Answer from the drawing. Dimensions are ordinates in mm from the lowest x, y and z of the part. Give positions to 0.01 mm unless a question says otherwise; leave off trailing zeros. Loops run counter-clockwise (first coordinate to the right, second up) from the corner with the lowest first, then second, coordinate; pieces in that order, holes last. Notation, with made-up numbers: (8.5, 10.25) -> (29.5, 10.25) arc R24 cw to (29.5, 32.25) -> close; hole circle Ø11 at (57.25, 20.5). An arc over 180 degrees is marked (long way). Answer as CSV lines item,"result". Start each with the question number.
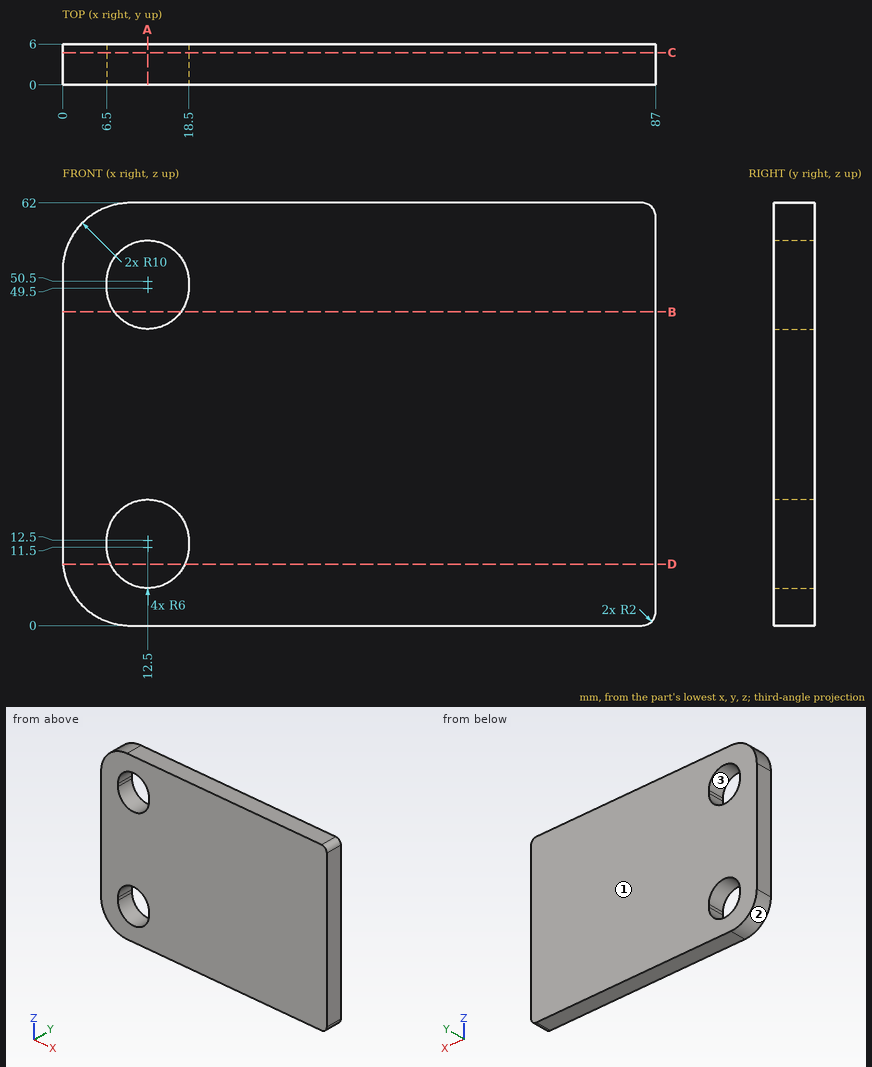
(1) Find section B-B on z = 46. Write down the section's boundary in (x, y), then the cut area to 3 significant figures.
(2) Find section A-A on x = 12.5. Write down the section's boundary in (y, z), then the cut area to 3 significant figures.
(3) Find section D-D on z = 9. Write down the section's boundary in (x, y).
(4) Find section C-C on y = 4.75. Write down the section's boundary in (x, z), then the cut area to 3 significant figures.
(5) Find the intervals of material crossed by line 1 along Z through (x, y) = (7.5, 2.25); line 2 along Z through (x, y) = (14, 3.9); line 3 along X through (y, z) = (0.55, 11), in increasing order. Write a range as from..to.
(6) The mould has two halves that part along Z. Classify the marked faces 1, 2 and 3: pulls with the +Z half, pulls with the -Z half, needs draft (parallel to the pull), parting line crosses it, or undercut.
Answer block:
1,outline,"(0, 0) -> (7.63, 0) -> (7.63, 6) -> (0, 6) -> close; (17.37, 0) -> (87, 0) -> (87, 6) -> (17.37, 6) -> close"
1,area,"464 mm2"
2,outline,"(0, 0) -> (6, 0) -> (6, 5.5) -> (0, 5.5) -> close; (0, 18.5) -> (6, 18.5) -> (6, 43.5) -> (0, 43.5) -> close; (0, 56.5) -> (6, 56.5) -> (6, 62) -> (0, 62) -> close"
2,area,"216 mm2"
3,outline,"(0.05, 0) -> (7.05, 0) -> (7.05, 6) -> (0.05, 6) -> close; (17.95, 0) -> (87, 0) -> (87, 6) -> (17.95, 6) -> close"
4,outline,"(0, 10) arc R10 ccw to (10, 0) -> (85, 0) arc R2 ccw to (87, 2) -> (87, 60) arc R2 ccw to (85, 62) -> (10, 62) arc R10 ccw to (0, 52) -> close; hole (6.5, 11.5) arc R6 ccw to (18.5, 11.5) -> (18.5, 12.5) arc R6 ccw to (6.5, 12.5) -> close; hole (6.5, 49.5) arc R6 ccw to (18.5, 49.5) -> (18.5, 50.5) arc R6 ccw to (6.5, 50.5) -> close"
4,area,"5,100 mm2"
5,line 1,"z = 0.32..8.18, 15.82..46.18, 53.82..61.68"
5,line 2,"z = 0..5.69, 18.31..43.69, 56.31..62"
5,line 3,"x = 0..6.52, 18.48..87"
6,face 1,"needs draft"
6,face 2,"pulls with the -Z half"
6,face 3,"undercut"
